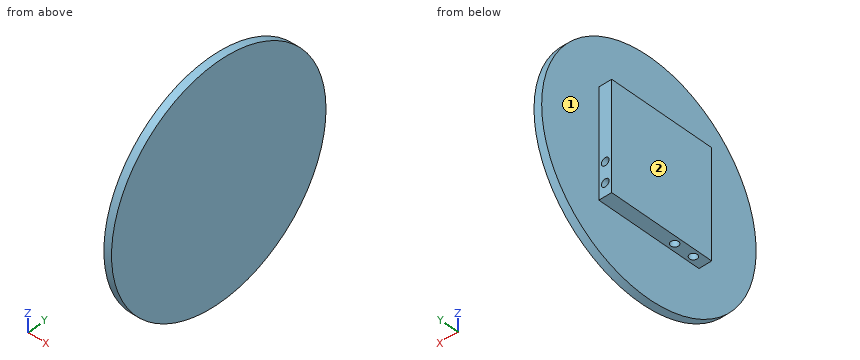
from build123d import *

# Parameters (mm, degrees)
F0_W            = 42
F0_H            = 42
F1_DEPTH        = 5
F2_R            = 1.5
F3_DEPTH        = 15
F3_COPIES_COUNT = 4
F5_R            = 45
F6_DEPTH        = 3


# Not quite as in the source:
# - a pattern or mirror of a feature is missing from the dataset's text; its kind, count and spacing are read off the source's solid


with BuildPart() as f1:
    # F0 (on Right) → F1 (new body)
    with BuildSketch(Plane.YZ):
        Rectangle(F0_W, F0_H)
    extrude(amount=F1_DEPTH)

    # F2 (on face) → F3 (cut)
    with BuildSketch(Plane.XZ.offset(21)):
        with Locations((2.5, 16)):
            Circle(F2_R)
        with Locations((2.5, 8.126)):
            Circle(F2_R)
    f3 = extrude(amount=-F3_DEPTH, mode=Mode.SUBTRACT)

    # F3_copies: F3 ×4 about axis
    f3_copies_axis = Axis((0, 0, 0), (1, 0, 0))
    for i in range(1, F3_COPIES_COUNT):
        add(f3.rotate(f3_copies_axis, i * 360 / F3_COPIES_COUNT), mode=Mode.SUBTRACT)

    # F5 (on face) → F6 (join)
    with BuildSketch(Plane.YZ.offset(5)):
        Circle(F5_R)
    extrude(amount=F6_DEPTH)


solid = f1.part
Check sheet for the modelled part. Datum: model origin and axes. Units: mm. Face numbers are marked on the shaded views. A direction names the side the tool comes from. Coordinates: 2 decimals unless noted, no trailing zeros. Loops run counter-clockwise (first coordinate to the right, second up) from the corner with the lowest first, then second, coordinate; pieces in that order, holes last. Notation, with made-up numbers: (60, 22.5) -> (73, 22.5) arc R15 cw to (73, 39.5) -> close; hole circle Ø9 at (5, 86). An arc over 180 degrees is marked (long way). Write item = value, one per line. Start each with the question number.
1. Section check A-A on y = 0. Record the cut outline in (x, z).
2. Section check D-D on z = 28.5. Record the cut outline in (x, y), then the cut area to 3 significant figures.
3. Depth check by flat-ended pin: P1, Ø2.5, axis at x = 3, z = 8, coming from the -Y side; P2, Ø0.9, axis at x = 2, y = 8, coming from the +Z side; P3, Ø1.5, axis at x = 3, y = -0.5, coming from the -Z side; P4, Ø12, axis at y = -24, z = 3.5, coming from the -X side. Enter the tip coordinate at first touch or a pass-through.
4. Section check C-C on y = -16. Record the cut outline in (x, z), then the cut area to 3 significant figures.
5. Material ranges on line 1 (Y direction, x = 2.5, z = -9); line 2 (Y direction, x = 2.5, z = 15.75); line 3 (Z direction, x = 2.75, y = 0.5), recorded low to high.
6. Tool access check on the marked faces 1 and 2. Record the directions out of +Z, -Z, +X, -X, +Y, -Y that give a thin tool (end or side, any length) a straight path to the whole face; none if there is none.
Responses:
q1.outline = (0, -21) -> (5, -21) -> (5, -45) -> (8, -45) -> (8, 45) -> (5, 45) -> (5, 21) -> (0, 21) -> close
q2.outline = (5, -34.82) -> (8, -34.82) -> (8, 34.82) -> (5, 34.82) -> close
q2.area = 209 mm2
q3.P1 = -21
q3.P2 = 6
q3.P3 = -21
q3.P4 = 0
q4.outline = (0, -21) -> (1, -21) -> (1, -6) -> (4, -6) -> (4, -21) -> (5, -21) -> (5, -42.06) -> (8, -42.06) -> (8, 42.06) -> (5, 42.06) -> (5, 21) -> (0, 21) -> close; hole circle Ø3 at (2.5, 8.13); hole circle Ø3 at (2.5, 16)
q4.area = 403 mm2
q5.line_1 = -21 to -17.5, -14.5 to -9.63, -6.63 to 6
q5.line_2 = -6 to 6.63, 9.63 to 14.5, 17.5 to 21
q5.line_3 = -21 to 21
q6.face_1 = -X
q6.face_2 = +Z, -Z, -X, +Y, -Y
